Model file for the job. Use its own axes, mm. Face numbers are marked on the shaded views. A direction names the side the tool comes from. Round coordinates to 2 decimals unless told otherwise and drop trailing zeros. Order: outer loops, then holes, each group sorted by start corner. A loop starts at its lowest first (then second) coordinate and runs counter-clockwise, first axis right, second up. Notation, with made-up numbers: (2.5, 44) - (45.5, 44) arc R19 cw to (45.5, 72) - close; hole circle Ø8 at (23, 43.25). An arc over 180 degrees is marked (long way). Use one line per item in the form item = value.
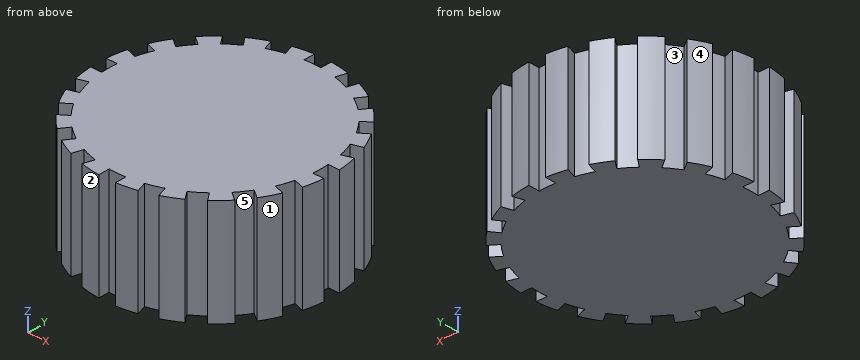
Autodesk Inventor part; units mm, degrees
ref_plane "YZ Plane" through (0, 0, 0) normal (1, 0, 0) x (0, 1, 0)
ref_plane "XZ Plane" through (0, 0, 0) normal (0, 1, 0) x (-1, 0, 0)
ref_plane "XY Plane" through (0, 0, 0) normal (0, 0, 1) x (1, 0, 0)
sketch "Boceto1" plane through (0, 0, 0) normal (0, 0, 1) x (1, 0, 0)
  circle A0 centre (0, 0) radius 21
  dimension "d0" = 42
extrude "Extrusión1" add sketch "Boceto1" along normal blind 19
sketch "Boceto2" plane through (0, 0, 19) normal (0, 0, 1) x (1, 0, 0)
  circle A0 centre (0, 0) radius 21 construction
  circle A1 centre (0, 0) radius 21
  circle A2 centre (0, 0) radius 19 construction
  arc A3 (1.5, 20.9464) -> (-1.5, 20.9464) centre (0, 0) ccw
  line L0 (1.5, 20.9464) -> (1.5, 18.9407)
  line L1 (-1.5, 20.9464) -> (-1.5, 18.9407)
  arc A4 (1.5, 18.9407) -> (-1.5, 18.9407) centre (0, 0) ccw
  arc A5 (7.8994, 19.4576) -> (5.0462, 20.3847) centre (0, 0) ccw
  line L2 (7.8994, 19.4576) -> (7.2796, 17.5501)
  line L3 (5.0462, 20.3847) -> (4.4264, 18.4772)
  arc A6 (7.2796, 17.5501) -> (4.4264, 18.4772) centre (0, 0) ccw
  arc A7 (13.5255, 16.0643) -> (11.0984, 17.8276) centre (0, 0) ccw
  line L4 (13.5255, 16.0643) -> (12.3466, 14.4417)
  line L5 (11.0984, 17.8276) -> (9.9195, 16.205)
  arc A8 (12.3466, 14.4417) -> (9.9195, 16.205) centre (0, 0) ccw
  arc A9 (17.8276, 11.0984) -> (16.0643, 13.5255) centre (0, 0) ccw
  line L6 (17.8276, 11.0984) -> (16.205, 9.9195)
  line L7 (16.0643, 13.5255) -> (14.4417, 12.3466)
  arc A10 (16.205, 9.9195) -> (14.4417, 12.3466) centre (0, 0) ccw
  arc A11 (20.3847, 5.0462) -> (19.4576, 7.8994) centre (0, 0) ccw
  line L8 (20.3847, 5.0462) -> (18.4772, 4.4264)
  line L9 (19.4576, 7.8994) -> (17.5501, 7.2796)
  arc A12 (18.4772, 4.4264) -> (17.5501, 7.2796) centre (0, 0) ccw
  arc A13 (20.9464, -1.5) -> (20.9464, 1.5) centre (0, 0) ccw
  line L10 (20.9464, -1.5) -> (18.9407, -1.5)
  line L11 (20.9464, 1.5) -> (18.9407, 1.5)
  arc A14 (18.9407, -1.5) -> (18.9407, 1.5) centre (0, 0) ccw
  arc A15 (19.4576, -7.8994) -> (20.3847, -5.0462) centre (0, 0) ccw
  line L12 (19.4576, -7.8994) -> (17.5501, -7.2796)
  line L13 (20.3847, -5.0462) -> (18.4772, -4.4264)
  arc A16 (17.5501, -7.2796) -> (18.4772, -4.4264) centre (0, 0) ccw
  arc A17 (16.0643, -13.5255) -> (17.8276, -11.0984) centre (0, 0) ccw
  line L14 (16.0643, -13.5255) -> (14.4417, -12.3466)
  line L15 (17.8276, -11.0984) -> (16.205, -9.9195)
  arc A18 (14.4417, -12.3466) -> (16.205, -9.9195) centre (0, 0) ccw
  arc A19 (11.0984, -17.8276) -> (13.5255, -16.0643) centre (0, 0) ccw
  line L16 (11.0984, -17.8276) -> (9.9195, -16.205)
  line L17 (13.5255, -16.0643) -> (12.3466, -14.4417)
  arc A20 (9.9195, -16.205) -> (12.3466, -14.4417) centre (0, 0) ccw
  arc A21 (5.0462, -20.3847) -> (7.8994, -19.4576) centre (0, 0) ccw
  line L18 (5.0462, -20.3847) -> (4.4264, -18.4772)
  line L19 (7.8994, -19.4576) -> (7.2796, -17.5501)
  arc A22 (4.4264, -18.4772) -> (7.2796, -17.5501) centre (0, 0) ccw
  arc A23 (-1.5, -20.9464) -> (1.5, -20.9464) centre (0, 0) ccw
  line L20 (-1.5, -20.9464) -> (-1.5, -18.9407)
  line L21 (1.5, -20.9464) -> (1.5, -18.9407)
  arc A24 (-1.5, -18.9407) -> (1.5, -18.9407) centre (0, 0) ccw
  arc A25 (-7.8994, -19.4576) -> (-5.0462, -20.3847) centre (0, 0) ccw
  line L22 (-7.8994, -19.4576) -> (-7.2796, -17.5501)
  line L23 (-5.0462, -20.3847) -> (-4.4264, -18.4772)
  arc A26 (-7.2796, -17.5501) -> (-4.4264, -18.4772) centre (0, 0) ccw
  arc A27 (-13.5255, -16.0643) -> (-11.0984, -17.8276) centre (0, 0) ccw
  line L24 (-13.5255, -16.0643) -> (-12.3466, -14.4417)
  line L25 (-11.0984, -17.8276) -> (-9.9195, -16.205)
  arc A28 (-12.3466, -14.4417) -> (-9.9195, -16.205) centre (0, 0) ccw
  arc A29 (-17.8276, -11.0984) -> (-16.0643, -13.5255) centre (0, 0) ccw
  line L26 (-17.8276, -11.0984) -> (-16.205, -9.9195)
  line L27 (-16.0643, -13.5255) -> (-14.4417, -12.3466)
  arc A30 (-16.205, -9.9195) -> (-14.4417, -12.3466) centre (0, 0) ccw
  arc A31 (-20.3847, -5.0462) -> (-19.4576, -7.8994) centre (0, 0) ccw
  line L28 (-20.3847, -5.0462) -> (-18.4772, -4.4264)
  line L29 (-19.4576, -7.8994) -> (-17.5501, -7.2796)
  arc A32 (-18.4772, -4.4264) -> (-17.5501, -7.2796) centre (0, 0) ccw
  arc A33 (-20.9464, 1.5) -> (-20.9464, -1.5) centre (0, 0) ccw
  line L30 (-20.9464, 1.5) -> (-18.9407, 1.5)
  line L31 (-20.9464, -1.5) -> (-18.9407, -1.5)
  arc A34 (-18.9407, 1.5) -> (-18.9407, -1.5) centre (0, 0) ccw
  arc A35 (-19.4576, 7.8994) -> (-20.3847, 5.0462) centre (0, 0) ccw
  line L32 (-19.4576, 7.8994) -> (-17.5501, 7.2796)
  line L33 (-20.3847, 5.0462) -> (-18.4772, 4.4264)
  arc A36 (-17.5501, 7.2796) -> (-18.4772, 4.4264) centre (0, 0) ccw
  arc A37 (-16.0643, 13.5255) -> (-17.8276, 11.0984) centre (0, 0) ccw
  line L34 (-16.0643, 13.5255) -> (-14.4417, 12.3466)
  line L35 (-17.8276, 11.0984) -> (-16.205, 9.9195)
  arc A38 (-14.4417, 12.3466) -> (-16.205, 9.9195) centre (0, 0) ccw
  arc A39 (-11.0984, 17.8276) -> (-13.5255, 16.0643) centre (0, 0) ccw
  line L36 (-11.0984, 17.8276) -> (-9.9195, 16.205)
  line L37 (-13.5255, 16.0643) -> (-12.3466, 14.4417)
  arc A40 (-9.9195, 16.205) -> (-12.3466, 14.4417) centre (0, 0) ccw
  arc A41 (-5.0462, 20.3847) -> (-7.8994, 19.4576) centre (0, 0) ccw
  line L38 (-5.0462, 20.3847) -> (-4.4264, 18.4772)
  line L39 (-7.8994, 19.4576) -> (-7.2796, 17.5501)
  arc A42 (-4.4264, 18.4772) -> (-7.2796, 17.5501) centre (0, 0) ccw
  point P0 (0, 21)
  point P1 (6.4894, 19.9722)
  point P2 (12.3435, 16.9894)
  point P3 (16.9894, 12.3435)
  point P4 (19.9722, 6.4894)
  point P5 (21, 0)
  point P6 (19.9722, -6.4894)
  point P7 (16.9894, -12.3435)
  point P8 (12.3435, -16.9894)
  point P9 (6.4894, -19.9722)
  point P10 (0, -21)
  point P11 (-6.4894, -19.9722)
  point P12 (-12.3435, -16.9894)
  point P13 (-16.9894, -12.3435)
  point P14 (-19.9722, -6.4894)
  point P15 (-21, 0)
  point P16 (-19.9722, 6.4894)
  point P17 (-16.9894, 12.3435)
  point P18 (-12.3435, 16.9894)
  point P19 (-6.4894, 19.9722)
  dimension "d3" = 38
  dimension "d4" = 3
  dimension "d7" = 360
extrude "Extrusión2" cut sketch "Boceto2" against normal through all contours A1 L10 A14 L11 | L8 A12 L9 A1 | A1 L12 A16 L13 | L6 A10 L7 A1 | A1 L14 A18 L15 | L4 A8 L5 A1 | A1 L16 A20 L17 | L2 A6 L3 A1 | A1 L18 A22 L19 | L0 A4 L1 A1 | A1 L20 A24 L21 | L38 A42 L39 A1 | A1 L22 A26 L23 | L36 A40 L37 A1 | A1 L24 A28 L25 | L34 A38 L35 A1 | A1 L26 A30 L27 | L32 A36 L33 A1 | A1 L28 A32 L29 | L30 A34 L31 A1
properties part number "Llanta" material "Goma"
(1) Slice it at B-B on x = 17. Give the cut face in (y, z), then the cut area to 3 significant figures.
Report:
outline = (-10.5, 0) - (10.5, 0) - (10.5, 19) - (-10.5, 19) - close
area = 399 mm2
(2) Pin check, flat tips, straight feed: pin 1 (2 mm diameter, centred on x = 20, z = 6.5, fed in from +Y); pin 2 (1.5 mm diameter, centred on y = -6.5, z = 3.5, fed in from +X); pin 3 (1 mm diameter, centred on y = -20.5, z = 6, fed in from +X). Stop position of each tip, or through.
Report:
pin_1 = 8.94
pin_2 = 18.11
pin_3 = 5.05
(3) Slice it at A-A on y = 1. Give the cut face in (x, z), then the cut area to 3 significant figures.
Report:
outline = (-18.97, 0) - (18.97, 0) - (18.97, 19) - (-18.97, 19) - close
area = 721 mm2
(4) Tool access for the marked faces 4 and 5: list every direction of +Z, -Z, +X, -X, +Y, -Y with a clear straight run to the whole face (end or side of a thin tool).
Report:
face_4 = +Z, -Z, -X, +Y
face_5 = +Z, -Z
(5) Pull direction X, two halves, no side cores. Call the marked faces 1, 2 and 3: released by +X, released by -X, zero draft, split by the parting line, or undercut.
Report:
face_1 = released by +X
face_2 = released by -X
face_3 = undercut
(6) Probe probe 1 along X at (y, z) = (-15, 7); probe 2 along X at (y, z) = (18.5, 9.25); probe 3 along X at (y, z) = (-0.5, 12.25). List the from-to ranges inside material, lowest first. Write a range as [from, to].
Report:
probe_1 = [-14.7, -12.75], [-11.66, 11.66], [12.75, 14.7]
probe_2 = [-9.94, -7.59], [-4.43, 4.43], [7.59, 9.94]
probe_3 = [-18.99, 18.99]
